Read the model definition and answer for the solid it produces. Units are mm, in the model's axes. A direction names the side the tool comes from. Coordinates: 2 decimals unless noted, no trailing zeros.
from build123d import *

# Parameters (mm, degrees)
BOSS_EXTRUDE1_DEPTH = 76.2
CUT_EXTRUDE1_DEPTH  = 1629.177643871
CUT_EXTRUDE2_DEPTH  = 1629.177644016
FILLET1_R           = 50.8
CUT_EXTRUDE3_DEPTH  = 48.26
CUT_EXTRUDE4_DEPTH  = 1506.588524386
SKETCH5_W           = 101.6
SKETCH5_H           = 127
CUT_EXTRUDE5_DEPTH  = 25.4
LPATTERN1_COUNT     = 2
LPATTERN1_PITCH     = 254
SKETCH6_W           = 304.8
SKETCH6_H           = 127
CUT_EXTRUDE6_DEPTH  = 153.67


with BuildPart() as part:
    # Sketch1 → Boss-Extrude1 (new, symmetric)
    with BuildSketch(Plane.XY):
        with BuildLine():
            Line((0, 0), (0, 381))
            Line((0, 381), (457.2, 1016))
            Line((457.2, 1016), (1270, 1016))
            Line((1270, 1016), (1270, 381))
            ThreePointArc((1270, 381), (1000.592316368, 269.407683632), (889, 0))
            Line((889, 0), (0, 0))
        make_face()
    extrude(amount=BOSS_EXTRUDE1_DEPTH, both=True)

    # Sketch2 → Cut-Extrude1 (cut, through all)
    with BuildSketch(Plane(origin=(1270, 0, 0), x_dir=(0, 0, -1), z_dir=(1, 0, 0))):
        with BuildLine():
            Line((-76.2, 1016), (38.1, 1016))
            add(Edge.make_bspline(
                [(38.1, 1016), (-59.769782928, 824.490487528), (-71.194008123, 596.511314057), (-76.2, 381)],
                knots=[0, 0, 0, 0, 1, 1, 1, 1], degree=3))
            Line((-76.2, 381), (-76.2, 1016))
        make_face()
    extrude(amount=-CUT_EXTRUDE1_DEPTH, mode=Mode.SUBTRACT)

    # Sketch3 → Cut-Extrude2 (cut, through all)
    with BuildSketch(Plane.ZY):
        with BuildLine():
            Line((76.2, 0), (12.7, 0))
            add(Edge.make_bspline(
                [(76.2, 381), (64.47102467, 274.36986488), (67.170280271, 132.109019993), (12.7, 0)],
                knots=[0, 0, 0, 0, 1, 1, 1, 1], degree=3))
            Line((76.2, 381), (76.2, 0))
        make_face()
    extrude(amount=-CUT_EXTRUDE2_DEPTH, mode=Mode.SUBTRACT)

    # Fillet1
    fillet1_edges = [part.edges().sort_by_distance(p)[0] for p in [
        (635, 381, 76.2),
    ]]
    fillet(fillet1_edges, radius=FILLET1_R)

    # Sketch4 → Cut-Extrude3 (cut)
    with BuildSketch(Plane(origin=(0, 0, -76.2), x_dir=(-1, 0, 0), z_dir=(0, 0, -1))):
        Polygon((-1208.685916752, 962.035600553), (-1208.685916752, 479.435600553), (-171.968106524, 479.435600553), (-497.485916752, 962.035600553), align=None)
    extrude(amount=-CUT_EXTRUDE3_DEPTH, mode=Mode.SUBTRACT)

    # 3DSketch1 → Cut-Extrude4 (cut, through all)
    with BuildSketch(Plane(origin=(1178.205916752, 931.555600553, -27.94), x_dir=(-0.9138470118423624, -0.4060586644153593, 0), z_dir=(0, 0, 1))):
        Polygon((0, 0), (171.210575264, 385.314454073), (1038.372129325, 0), (607.263673126, -269.831462884), align=None)
    extrude(amount=CUT_EXTRUDE4_DEPTH, mode=Mode.SUBTRACT)

    # Sketch5 → Cut-Extrude5 (cut)
    with BuildSketch(Plane(origin=(-180.663856691, 130.077976818, 0), x_dir=(0, 0, 1), z_dir=(-0.8115343414514944, 0.5843047258450759, 0))):
        with Locations((-25.4, 448.894584093)):
            Rectangle(SKETCH5_W, SKETCH5_H)
    cut_extrude5 = extrude(amount=-CUT_EXTRUDE5_DEPTH, mode=Mode.SUBTRACT)

    # LPattern1: Cut-Extrude5 ×2
    with Locations(*[Vector(0.5843047258450755, 0.8115343414514946, 0) * (i * LPATTERN1_PITCH) for i in range(1, LPATTERN1_COUNT)]):
        add(cut_extrude5, mode=Mode.SUBTRACT)

    # Sketch6 → Cut-Extrude6 (cut)
    with BuildSketch(Plane.XY.offset(128.348177056)):
        with Locations((735.261288267, 372.214025497)):
            Rectangle(SKETCH6_W, SKETCH6_H)
    extrude(amount=-CUT_EXTRUDE6_DEPTH, mode=Mode.SUBTRACT)


solid = part.part
Q1. Straight lines are drawn through the part: probe 1 along Y at (x, z) = (650.5, -13); probe 2 along Z at (x, y) = (1176, 399.5); probe 3 along Y at (x, z) = (748, 5). For each, find the intervals that lie inside material, in ascending order.
Findings below:
probe 1: y = 0 to 308.71, 435.71 to 509.92, 931.56 to 961.73
probe 2: z = -76.2 to 75.75
probe 3: y = 0 to 308.71, 435.71 to 509.92
Q2. Which of the six approach directions +Z, -Z, +X, -X, +Y, -Y give full straight-line access (tool end or side, diameter ignored) to faces 5 (the face through (841, 931.556, -15)), 6 (the face through (858, 1016, -57)), 7 (the face through (887.661, 371, 26)), 8 (the face through (332.45, 717.36, -52.41))?
Findings below:
face 5: +Z, -Z
face 6: +Z, -Z, +X, -X, +Y
face 7: +Z
face 8: -Z
Q3. Determine the mould class of faces 1 (the face through (582.861, 371, 26)), 2 (the face through (770, 507, -27.94)), 3 (the face through (174.6, 623.5, 1)), 4 (the face through (451, 0, -31)) for opening direction X: +X half, -X half, draft (parallel to the pull), parting line (faces both ways), or undercut.
Findings below:
face 1: undercut
face 2: undercut
face 3: -X half
face 4: draft
Q4. Flat-ended cylindrical pins translate along their axes: pin 1 Ø2 at (x, z) = (881.5, -12) entering from +Y; pin 2 Ø5 at (x, y) = (767, 391.5) entering from +Z; pin 3 Ø6 at (y, z) = (510.5, -48.5) entering from -X. Find the tip coordinate at first contact, or state that the pin passes through.
Findings below:
pin 1: stops at y = 961.73
pin 2: stops at z = -25.32
pin 3: stops at x = 122.38
